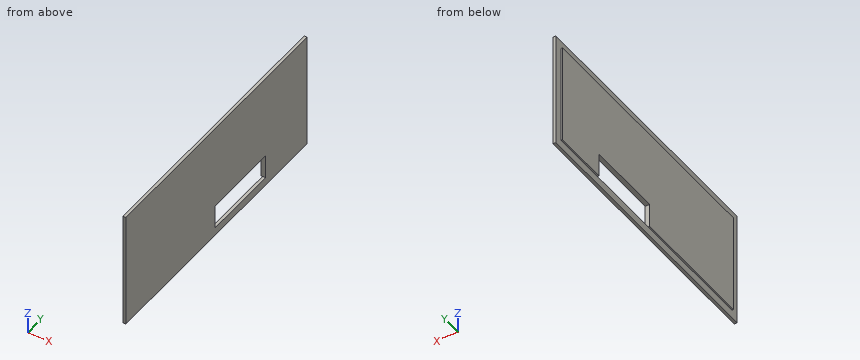
```python
from build123d import *

# Parameters (mm, degrees)
SKETCH_1_W          = 95
SKETCH_1_H          = 38.85
EXTRUDE_1_DEPTH     = 1
SKETCH_2_W          = 33.45
SKETCH_2_H          = 89.6
EXTRUDE_2_DEPTH     = 0.5
SKETCH_3_W          = 7.954176302
SKETCH_3_H          = 26.586882205
CUT_EXTRUDE_1_DEPTH = 2


with BuildPart() as part:
    # Эскиз1 → Бобышка-Вытянуть1 (new body)
    with BuildSketch(Plane(origin=(0.5, 0, 0), x_dir=(0, -1, 0), z_dir=(-1, 0, 0))):
        with Locations((-53.35, 22.825)):
            Rectangle(SKETCH_1_W, SKETCH_1_H)
    extrude(amount=-EXTRUDE_1_DEPTH)

    # Эскиз2 → Бобышка-Вытянуть2 (add)
    with BuildSketch(Plane.ZY.offset(-0.5)):
        with Locations((22.825, 53.35)):
            Rectangle(SKETCH_2_W, SKETCH_2_H)
    extrude(amount=EXTRUDE_2_DEPTH)

    # Эскиз3 → Вырез-Вытянуть1 (cut)
    with BuildSketch(Plane.ZY):
        with Locations((10.077088151, 65.780778583)):
            Rectangle(SKETCH_3_W, SKETCH_3_H)
    extrude(amount=-CUT_EXTRUDE_1_DEPTH, mode=Mode.SUBTRACT)


solid = part.part
```
Check sheet for the modelled part. Datum: model origin and axes. Units: mm. Round coordinates to 2 decimals unless told otherwise and drop trailing zeros. Order: outer loops, then holes, each group sorted by start corner. A loop starts at its lowest first (then second) coordinate and runs counter-clockwise, first axis right, second up.
1) Section check A-A (y = 66). Record the boundary of the cut face in (x, z).
2) Section check C-C (x = 0.9). Record the boundary of the cut face in (y, z).
3) Section check D-D (z = 17.5). Record the boundary of the cut face in (x, y), and give its area (3 significant figures).
4) Go/stop test with flat-tipped pins: pin 1 Ø0.6 at (x, y) = (0, 30.5) entering from -Z; pin 2 Ø11.5 at (y, z) = (59, 26) entering from -X. Record where each tip stops, or that it passes through.
5) Scan lines: line 1 (Y direction, x = 0.65, z = 9.5); line 2 (Z direction, x = 0.8, y = 59); line 3 (Z direction, x = 0.45, y = 82). Record each from-to range of solid material in increasing order.
6) Section check B-B (z = 11.5). Record the boundary of the cut face in (x, y).
Result:
1. outline: (0, 14.05) - (1.5, 14.05) - (1.5, 42.25) - (0.5, 42.25) - (0.5, 39.55) - (0, 39.55) - close; (0.5, 3.4) - (1.5, 3.4) - (1.5, 6.1) - (0.5, 6.1) - close
2. outline: (5.85, 3.4) - (100.85, 3.4) - (100.85, 42.25) - (5.85, 42.25) - close; hole (52.49, 6.1) - (79.07, 6.1) - (79.07, 14.05) - (52.49, 14.05) - close
3. outline: (0, 8.55) - (0.5, 8.55) - (0.5, 5.85) - (1.5, 5.85) - (1.5, 100.85) - (0.5, 100.85) - (0.5, 98.15) - (0, 98.15) - close
3. area: 140 mm2
4. pin 1: stops at z = 6.1
4. pin 2: stops at x = 0
5. line 1: y = 5.85 to 52.49, 79.07 to 100.85
5. line 2: z = 3.4 to 6.1, 14.05 to 42.25
5. line 3: z = 6.1 to 39.55
6. outline: (0, 8.55) - (0.5, 8.55) - (0.5, 5.85) - (1.5, 5.85) - (1.5, 52.49) - (0, 52.49) - close; (0, 79.07) - (1.5, 79.07) - (1.5, 100.85) - (0.5, 100.85) - (0.5, 98.15) - (0, 98.15) - close
